Design review of the part shown in the three views and the two pictorial views. Dimensions are in mm from the part's minimum x, y and z. A direction names the side the tool comes from. Coordinates: 2 decimals unless noted, no trailing zeros. Write each loop counter-clockwise with the first axis right and the second up, starting at its lowest first coordinate (ties: lowest second). Pieces come first, ordered by that corner, then holes. Notation, with made-up numbers: M -6.75,17.5 L 21.25,17.5 A16 cw 21.25,25.5 Z; hole C 59.25,18.25 d1. An arc over 180 degrees is marked long. One line per question, with ' | ' between items.
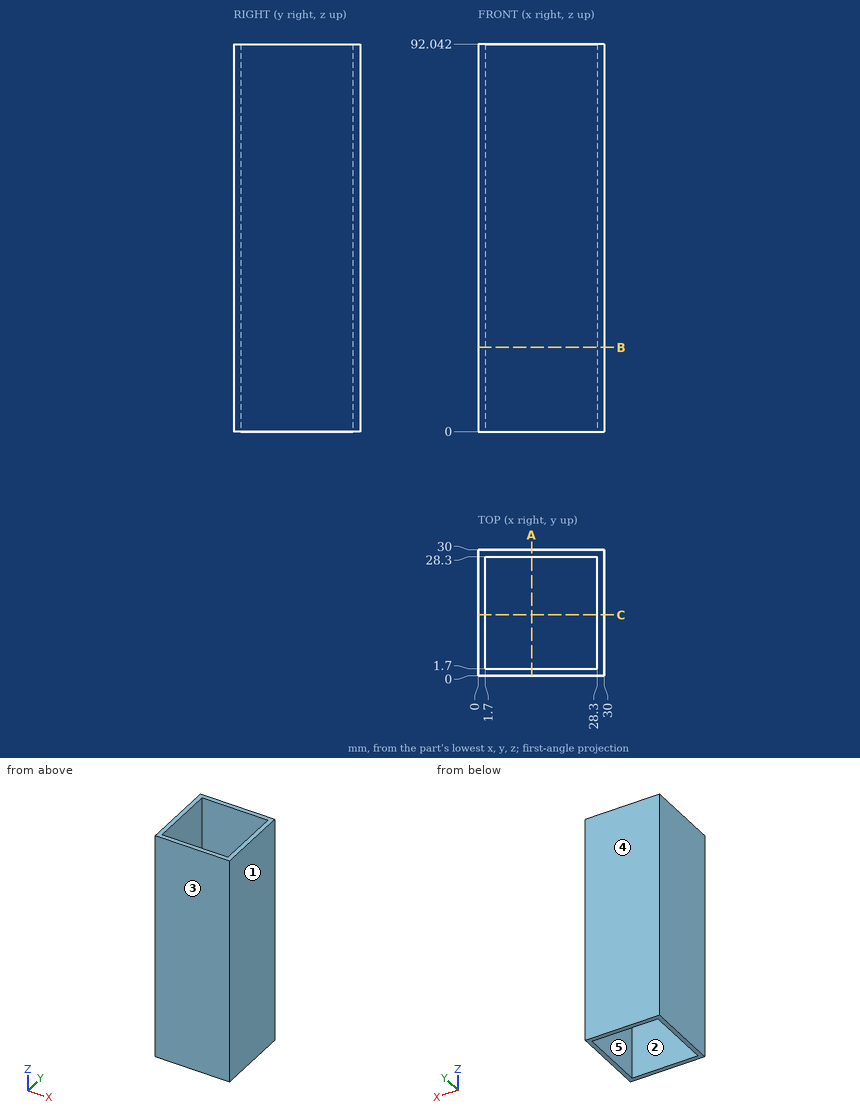
1. For line 1 along X through (y, z) = (6, 48.5), list the stretches that pass through material, from the lowest coordinate up.
Computed values:
line 1: x = 0 to 1.7, 28.3 to 30
2. Draft analysis for pull direction Y (two halves, no side actions). For the marked faces 3, 4 and 5, state which applies: pulls with the +Y half, pulls with the -Y half, needs draft (parallel to the pull), parting line crosses it, or undercut.
Computed values:
face 3: pulls with the -Y half | face 4: pulls with the +Y half | face 5: undercut
3. Take a section at A-A on x = 12.75. State the section outline as (y, z) points, plus the area to 3 significant figures.
Computed values:
outline: M 0,0 L 1.7,0 L 1.7,92.04 L 0,92.04 Z; M 28.3,0 L 30,0 L 30,92.04 L 28.3,92.04 Z | area: 313 mm2
4. Clearance check with a flat-ended pin moving along its axis: P1, Ø6, axis at x = 11.5, y = 23.5, coming from the -Z side. State where the tip first meets the part, or that it passes through.
Computed values:
P1: passes through
5. Machinability: for the marked faces 1 and 2, which of the approach directions +Z, -Z, +X, -X, +Y, -Y give a long, thin tool a straight path to every point of the face, cutting with its end or side? Answer none if there is none.
Computed values:
face 1: +Z, -Z, +X, +Y, -Y | face 2: +Z, -Z
6. Take a section at B-B on z = 20. State the section outline as (x, y) points.
Computed values:
outline: M 0,0 L 30,0 L 30,30 L 0,30 Z; hole M 1.7,1.7 L 28.3,1.7 L 28.3,28.3 L 1.7,28.3 Z
